Geometry: final body of the model. Coordinates: model frame, mm. Face numbers are marked on the shaded views. A direction names the side the tool comes from. Give positions to 0.01 mm unless a question says otherwise; leave off trailing zeros. Loops run counter-clockwise (first coordinate to the right, second up) from the corner with the lowest first, then second, coordinate; pieces in that order, holes last. Notation, with made-up numbers: (64.5, 13.5) -> (119.5, 13.5) arc R24 cw to (119.5, 48.5) -> close; hole circle Ø8 at (67, -27.5). An arc over 180 degrees is marked (long way). Answer in a Markdown table with one row per item. Add a question column.
1) Access query for the marked faces 5, 6 and 7. Directions: +Z, -Z, +X, -X, +Y, -Y. A direction counts if a zero-diameter tool reaches every point of the face in a straight line with its end or side. Return the directions, or none.
2) Section query C-C (y = -40). Return the cut outline in (x, z).
3) Line query: line 1 (Y direction, x = 10, z = -1.75); line 2 (X direction, y = -13, z = 3.5); line 3 (X direction, y = -19, z = -1.75). Output: solid intervals per line, ascending. Write a range as from..to.
4) Section query A-A (x = 8.25). Return the cut outline in (y, z).
5) Section query B-B (z = 0). Give the number of separate pieces and of enclosed holes in the cut face, plus the area to 3 significant figures.
6) First-contact query: P1, Ø12, axis at x = -5, y = -28, coming from the +Z side; P2, Ø6, axis at y = -31.5, z = 3, coming from the +X side; P3, Ø8, axis at x = 8.5, y = -27, coming from the +Z side. Flat tips, straight axial feed; report the tip coordinate or a pass-through.
7) Draft query along Y for the marked faces 1, 2, 3 and 4. Return one class per face: +Y half, -Y half, draft (parallel to the pull), parting line (faces both ways), or undercut.
```python
from build123d import *

# Parameters (mm, degrees)
SKETCH1_R                = 1.6
BOSS_EXTRUDE1_DEPTH      = 2.3
SKETCH2_R                = 5.765
BOSS_EXTRUDE2_DEPTH      = 7.7
SKETCH3_W                = 13
SKETCH3_H                = 26.5
BOSS_EXTRUDE3_DEPTH      = 5.75
BOSS_EXTRUDE3_DEPTH_BACK = 5.75
SKETCH4_W                = 1
SKETCH4_H                = 6
CHAMFER1_SIZE            = 3
FILLET1_R                = 3
CHAMFER2_SIZE            = 0.3
SKETCH9_R                = 2.25
CUT_EXTRUDE1_DEPTH       = 0.2
CUT_EXTRUDE2_DEPTH       = 1
SKETCH11_R               = 2.25
SKETCH11_R_2             = 2.15
CUT_EXTRUDE3_DEPTH       = 0.5
FILLET2_R                = 0.2
SKETCH12_R               = 0.3
CUT_EXTRUDE4_DEPTH       = 1
BOSS_EXTRUDE4_DEPTH      = 1


with BuildPart() as part:
    # Sketch1 → Boss-Extrude1 (new body)
    with BuildSketch(Plane(origin=(0, 0, 0), x_dir=(1, 0, 0), z_dir=(0, 1, 0))):
        with BuildLine():
            Line((3, 5.765), (-3, 5.765))
            Line((-3, 5.765), (-10.043565082, 3.861472766))
            ThreePointArc((-10.043565082, 3.861472766), (-13, 0), (-10.043565082, -3.861472766))
            Line((-10.043565082, -3.861472766), (-3, -5.765))
            Line((-3, -5.765), (3, -5.765))
            Line((3, -5.765), (10.043565082, -3.861472766))
            ThreePointArc((10.043565082, -3.861472766), (13, 0), (10.043565082, 3.861472766))
            Line((10.043565082, 3.861472766), (3, 5.765))
        make_face()
        with Locations((9, 0)):
            Circle(SKETCH1_R, mode=Mode.SUBTRACT)
        with Locations((-9, 0)):
            Circle(SKETCH1_R, mode=Mode.SUBTRACT)
    extrude(amount=-BOSS_EXTRUDE1_DEPTH)

    # Sketch2 → Boss-Extrude2 (add)
    with BuildSketch(Plane.XZ.offset(2.3)):
        Circle(SKETCH2_R)
    extrude(amount=BOSS_EXTRUDE2_DEPTH)

    # Sketch3 → Boss-Extrude3 (add, two sides)
    with BuildSketch(Plane.XY) as boss_extrude3_sk:
        with Locations((0, -23.25)):
            Rectangle(SKETCH3_W, SKETCH3_H)
    extrude(amount=BOSS_EXTRUDE3_DEPTH)
    extrude(boss_extrude3_sk.sketch, amount=-BOSS_EXTRUDE3_DEPTH_BACK)

    # Sketch4 → Revolve1 (revolve)
    with BuildSketch(Plane.XY):
        with Locations((0.5, -39.5)):
            Rectangle(SKETCH4_W, SKETCH4_H)
    revolve(axis=Axis((0, -36.5, 0), (0, -1, 0)))

    # Chamfer1
    chamfer1_edges = [part.edges().sort_by_distance(p)[0] for p in [
        (-6.5, -36.5, 0),
        (0, -36.5, -5.75),
        (6.5, -36.5, 0),
        (0, -36.5, 5.75),
    ]]
    chamfer(chamfer1_edges, length=CHAMFER1_SIZE)

    # Fillet1
    fillet1_edges = [part.edges().sort_by_distance(p)[0] for p in [
        (-6.5, -21.75, 5.75),
        (6.5, -21.75, 5.75),
    ]]
    fillet(fillet1_edges, radius=FILLET1_R)

    # Chamfer2
    chamfer2_edges = [part.edges().sort_by_distance(p)[0] for p in [
        (-1, -42.5, 0),
    ]]
    chamfer(chamfer2_edges, length=CHAMFER2_SIZE)

    # Sketch9 → Cut-Extrude1 (cut)
    with BuildSketch(Plane(origin=(0, 0, 0), x_dir=(1, 0, 0), z_dir=(0, 1, 0))):
        Circle(SKETCH9_R)
        Polygon((0, 1.5011107), (-1.3, 0.75055535), (-1.3, -0.75055535), (0, -1.5011107), (1.3, -0.75055535), (1.3, 0.75055535), align=None, mode=Mode.SUBTRACT)
    extrude(amount=-CUT_EXTRUDE1_DEPTH, mode=Mode.SUBTRACT)

    # Sketch10 → Cut-Extrude2 (cut)
    with BuildSketch(Plane(origin=(0, 0, 0), x_dir=(1, 0, 0), z_dir=(0, 1, 0))):
        Polygon((1.3, 0.75055535), (0, 1.5011107), (-1.3, 0.75055535), (-1.3, -0.75055535), (0, -1.5011107), (1.3, -0.75055535), align=None)
    extrude(amount=-CUT_EXTRUDE2_DEPTH, mode=Mode.SUBTRACT)

    # Sketch11 → Cut-Extrude3 (cut)
    with BuildSketch(Plane(origin=(0, -0.2, 0), x_dir=(1, 0, 0), z_dir=(0, 1, 0))):
        Circle(SKETCH11_R)
        Circle(SKETCH11_R_2, mode=Mode.SUBTRACT)
    extrude(amount=-CUT_EXTRUDE3_DEPTH, mode=Mode.SUBTRACT)

    # Fillet2
    fillet2_edges = [part.edges().sort_by_distance(p)[0] for p in [
        (-2.15, -0.2, 0),
    ]]
    fillet(fillet2_edges, radius=FILLET2_R)

    # Sketch12 → Cut-Extrude4 (cut)
    with BuildSketch(Plane(origin=(0, 0, -5.75), x_dir=(-1, 0, 0), z_dir=(0, 0, -1))):
        with Locations((0, -32.5)):
            Circle(SKETCH12_R)
        with BuildLine():
            Line((-6.5, -11), (6.5, -11))
            Line((6.5, -11), (6.5, -33))
            Line((6.5, -33), (1, -33))
            Line((1, -33), (1, -32.5))
            ThreePointArc((1, -32.5), (0, -31.5), (-1, -32.5))
            Line((-1, -32.5), (-1, -33))
            Line((-1, -33), (-6.5, -33))
            Line((-6.5, -33), (-6.5, -11))
        make_face()
    extrude(amount=-CUT_EXTRUDE4_DEPTH, mode=Mode.SUBTRACT)

    # Sketch13 → Boss-Extrude4 (add)
    with BuildSketch(Plane(origin=(0, 0, -4.75), x_dir=(-1, 0, 0), z_dir=(0, 0, -1))):
        with BuildLine():
            Line((6.4, -11.1), (-6.4, -11.1))
            Line((-6.4, -11.1), (-6.4, -32.9))
            Line((-6.4, -32.9), (-1.1, -32.9))
            Line((-1.1, -32.9), (-1.1, -32.5))
            ThreePointArc((-1.1, -32.5), (0, -31.4), (1.1, -32.5))
            Line((1.1, -32.5), (1.1, -32.9))
            Line((1.1, -32.9), (6.4, -32.9))
            Line((6.4, -32.9), (6.4, -11.1))
        make_face()
    extrude(amount=BOSS_EXTRUDE4_DEPTH)


solid = part.part
```
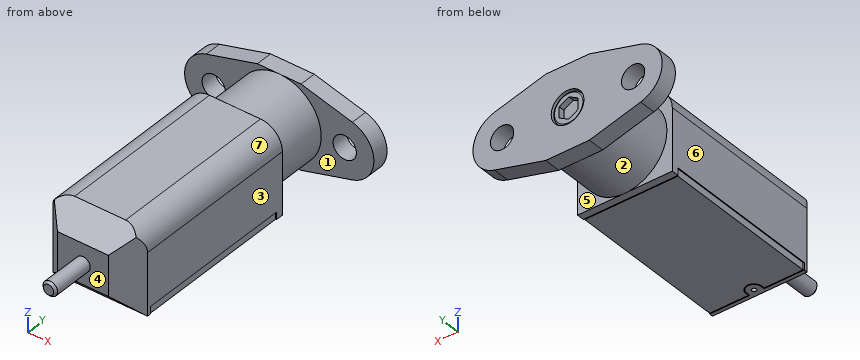
Evaluation:
| question | item | result |
|---|---|---|
| 1 | face 5 | +X |
| 1 | face 6 | +Z, -Z, -X, -Y |
| 1 | face 7 | +Z, +X, -Y |
| 2 | outline | circle Ø2 at (0, 0) |
| 3 | line 1 | -2.3..0 |
| 3 | line 2 | -6.4..6.4 |
| 3 | line 3 | -6.5..6.5 |
| 4 | outline | (-2.3, -4.35) -> (0, -4.35) -> (0, -1.41) -> (-2.3, -1.41) -> close; (-2.3, 1.41) -> (0, 1.41) -> (0, 4.35) -> (-2.3, 4.35) -> close |
| 5 | separate pieces | 3 |
| 5 | enclosed holes | 0 |
| 5 | area | 478 mm² |
| 6 | P1 | z = 5.75 |
| 6 | P2 | x = 6.5 |
| 6 | P3 | z = 5.58 |
| 7 | face 1 | undercut |
| 7 | face 2 | undercut |
| 7 | face 3 | draft |
| 7 | face 4 | -Y half |
